For this review, take the finished solid that the model builds, in its own axes (mm). A direction names the side the tool comes from. Coordinates: 2 decimals unless noted, no trailing zeros. Loops run counter-clockwise (first coordinate to the right, second up) from the corner with the lowest first, then second, coordinate; pieces in that order, holes last. Notation, with made-up numbers: (67, 39) -> (73, 39) arc R12 cw to (73, 61) -> close; hole circle Ø4 at (45.25, 34). An arc over 180 degrees is marked (long way). Answer in a Markdown table with one row per item.
from build123d import *

# Parameters (mm, degrees)
BOSS_EXTRUDE1_DEPTH = 5.08
SKETCH2_R           = 2.54
CUT_EXTRUDE1_DEPTH  = 341.814621752
SKETCH3_R           = 2.54
CUT_EXTRUDE2_DEPTH  = 341.814621752
SKETCH4_W           = 3.81
SKETCH4_H           = 37.084
BOSS_EXTRUDE2_DEPTH = 11.43
SKETCH5_W           = 12.7
SKETCH5_H           = 2.54
BOSS_EXTRUDE3_DEPTH = 2.54
BOSS_EXTRUDE4_START = 2.54
SKETCH6_R           = 5.08
SKETCH6_R_2         = 2.54
BOSS_EXTRUDE4_DEPTH = 2.54
SKETCH7_W           = 5.08
SKETCH7_H           = 101.6
BOSS_EXTRUDE5_DEPTH = 57.15
CUT_EXTRUDE3_REACH  = 257.636
SKETCH8_R           = 1.905
SKETCH8_R_2         = 2.54
CUT_EXTRUDE5_REACH  = 257.636
SKETCH10_R          = 2.54
CUT_EXTRUDE7_DEPTH  = 25.4
CUT_EXTRUDE8_DEPTH  = 25.4
CUT_EXTRUDE9_DEPTH  = 346.535703654
SKETCH15_R          = 2.413
SKETCH15_R_2        = 2.54
CUT_EXTRUDE10_DEPTH = 256.636204987


with BuildPart() as part:
    # Sketch1 → Boss-Extrude1 (new body)
    with BuildSketch(Plane(origin=(0, 0, 0), x_dir=(1, 0, 0), z_dir=(0, 1, 0))):
        Polygon((0, 0), (254, 0), (304.8, 76.2), (254, 152.4), (0, 152.4), align=None)
    extrude(amount=BOSS_EXTRUDE1_DEPTH)

    # Sketch2 → Cut-Extrude1 (cut, through all)
    with BuildSketch(Plane(origin=(0, 5.08, 0), x_dir=(1, 0, 0), z_dir=(0, 1, 0))):
        with Locations(Location((76.2, 38.7985, 0), (0, 0, 270))):
            Circle(SKETCH2_R)
        with Locations(Location((167.64, 38.7985, 0), (0, 0, 270))):
            Circle(SKETCH2_R)
        with Locations(Location((167.64, 113.6015, 0), (0, 0, 90))):
            Circle(SKETCH2_R)
        with Locations(Location((76.2, 113.6015, 0), (0, 0, 90))):
            Circle(SKETCH2_R)
    extrude(amount=-CUT_EXTRUDE1_DEPTH, mode=Mode.SUBTRACT)

    # Sketch3 → Cut-Extrude2 (cut, through all)
    with BuildSketch(Plane(origin=(0, 5.08, 0), x_dir=(1, 0, 0), z_dir=(0, 1, 0))):
        with Locations(Location((279.4, 68.58, 0), (0, 0, 270))):
            Circle(SKETCH3_R)
        with Locations(Location((279.4, 83.82, 0), (0, 0, 90))):
            Circle(SKETCH3_R)
    extrude(amount=-CUT_EXTRUDE2_DEPTH, mode=Mode.SUBTRACT)

    # Sketch4 → Boss-Extrude2 (add)
    with BuildSketch(Plane(origin=(0, 5.08, 0), x_dir=(1, 0, 0), z_dir=(0, 1, 0))):
        with Locations((42.545, 18.542)):
            Rectangle(SKETCH4_W, SKETCH4_H)
        with Locations((59.055, 18.542)):
            Rectangle(SKETCH4_W, SKETCH4_H)
        with Locations((59.055, 133.858)):
            Rectangle(SKETCH4_W, SKETCH4_H)
        with Locations((42.545, 133.858)):
            Rectangle(SKETCH4_W, SKETCH4_H)
    extrude(amount=BOSS_EXTRUDE2_DEPTH)

    # Sketch5 → Boss-Extrude3 (add)
    with BuildSketch(Plane(origin=(0, 5.08, 0), x_dir=(1, 0, 0), z_dir=(0, 1, 0))):
        with Locations((50.8, 1.27)):
            Rectangle(SKETCH5_W, SKETCH5_H)
        with Locations((50.8, 151.13)):
            Rectangle(SKETCH5_W, SKETCH5_H)
        with Locations((50.8, 116.586)):
            Rectangle(SKETCH5_W, SKETCH5_H)
        with Locations((50.8, 35.814)):
            Rectangle(SKETCH5_W, SKETCH5_H)
    extrude(amount=BOSS_EXTRUDE3_DEPTH)

    # Sketch6 → Boss-Extrude4 (add)
    # profile 1 of 4: a face of its own
    with BuildSketch(Plane(origin=(0, 5.08, 0), x_dir=(1, 0, 0), z_dir=(0, 1, 0)).offset(BOSS_EXTRUDE4_START)):
        with Locations(Location((76.2, 38.7985, 0), (0, 0, 90))):
            Circle(SKETCH6_R)
        with Locations(Location((76.2, 38.7985, 0), (0, 0, 270))):
            Circle(SKETCH6_R_2, mode=Mode.SUBTRACT)
    # profile 2 of 4: a face of its own
    with BuildSketch(Plane(origin=(0, 5.08, 0), x_dir=(1, 0, 0), z_dir=(0, 1, 0)).offset(BOSS_EXTRUDE4_START)):
        with Locations(Location((167.64, 38.7985, 0), (0, 0, 90))):
            Circle(SKETCH6_R)
        with Locations(Location((167.64, 38.7985, 0), (0, 0, 270))):
            Circle(SKETCH6_R_2, mode=Mode.SUBTRACT)
    # profile 3 of 4: a face of its own
    with BuildSketch(Plane(origin=(0, 5.08, 0), x_dir=(1, 0, 0), z_dir=(0, 1, 0)).offset(BOSS_EXTRUDE4_START)):
        with Locations(Location((167.64, 113.6015, 0), (0, 0, 90))):
            Circle(SKETCH6_R)
        with Locations(Location((167.64, 113.6015, 0), (0, 0, 270))):
            Circle(SKETCH6_R_2, mode=Mode.SUBTRACT)
    # profile 4 of 4: a face of its own
    with BuildSketch(Plane(origin=(0, 5.08, 0), x_dir=(1, 0, 0), z_dir=(0, 1, 0)).offset(BOSS_EXTRUDE4_START)):
        with Locations(Location((76.2, 113.6015, 0), (0, 0, 90))):
            Circle(SKETCH6_R)
        with Locations(Location((76.2, 113.6015, 0), (0, 0, 90))):
            Circle(SKETCH6_R_2, mode=Mode.SUBTRACT)
    extrude(amount=-BOSS_EXTRUDE4_DEPTH)

    # Sketch7 → Boss-Extrude5 (add)
    with BuildSketch(Plane(origin=(0, 5.08, 0), x_dir=(1, 0, 0), z_dir=(0, 1, 0))):
        with Locations((193.04, 76.2)):
            Rectangle(SKETCH7_W, SKETCH7_H)
    extrude(amount=BOSS_EXTRUDE5_DEPTH)

    # Sketch8 → Cut-Extrude3 (cut, up to next)
    with BuildSketch(Plane(origin=(195.58, 0, 0), x_dir=(0, 0, -1), z_dir=(1, 0, 0)), mode=Mode.PRIVATE) as cut_extrude3_sk1:
        with Locations((31.75, 55.88)):
            Circle(SKETCH8_R)
    cut_extrude3_tool1 = extrude(cut_extrude3_sk1.sketch, amount=-CUT_EXTRUDE3_REACH, mode=Mode.PRIVATE) & part.part
    # Sketch8 → Cut-Extrude3 (cut, up to next)
    with BuildSketch(Plane(origin=(195.58, 0, 0), x_dir=(0, 0, -1), z_dir=(1, 0, 0)), mode=Mode.PRIVATE) as cut_extrude3_sk2:
        with Locations((68.834, 55.88)):
            Circle(SKETCH8_R)
    cut_extrude3_tool2 = extrude(cut_extrude3_sk2.sketch, amount=-CUT_EXTRUDE3_REACH, mode=Mode.PRIVATE) & part.part
    # Sketch8 → Cut-Extrude3 (cut, up to next)
    with BuildSketch(Plane(origin=(195.58, 0, 0), x_dir=(0, 0, -1), z_dir=(1, 0, 0)), mode=Mode.PRIVATE) as cut_extrude3_sk3:
        with Locations((50.292, 40.64)):
            Circle(SKETCH8_R_2)
    cut_extrude3_tool3 = extrude(cut_extrude3_sk3.sketch, amount=-CUT_EXTRUDE3_REACH, mode=Mode.PRIVATE) & part.part
    add(cut_extrude3_tool1.solids().sort_by_distance((195.58, 55.88, -31.75))[0], mode=Mode.SUBTRACT)
    add(cut_extrude3_tool2.solids().sort_by_distance((195.58, 55.88, -68.834))[0], mode=Mode.SUBTRACT)
    add(cut_extrude3_tool3.solids().sort_by_distance((195.58, 40.64, -50.292))[0], mode=Mode.SUBTRACT)

    # Sketch10 → Cut-Extrude5 (cut, up to next)
    with BuildSketch(Plane(origin=(195.58, 0, 0), x_dir=(0, 0, -1), z_dir=(1, 0, 0)), mode=Mode.PRIVATE) as cut_extrude5_sk1:
        with Locations((76.2, 16.51)):
            Circle(SKETCH10_R)
    cut_extrude5_tool1 = extrude(cut_extrude5_sk1.sketch, amount=-CUT_EXTRUDE5_REACH, mode=Mode.PRIVATE) & part.part
    add(cut_extrude5_tool1.solids().sort_by_distance((195.58, 16.51, -76.2))[0], mode=Mode.SUBTRACT)

    # Sketch12 → Cut-Extrude7 (cut)
    with BuildSketch(Plane.ZY.offset(-40.64)):
        with BuildLine():
            Line((-20.447, 14.732), (-16.637, 14.732))
            ThreePointArc((-16.637, 14.732), (-15.875, 13.97), (-16.637, 13.208))
            Line((-16.637, 13.208), (-20.447, 13.208))
            ThreePointArc((-20.447, 13.208), (-21.209, 13.97), (-20.447, 14.732))
        make_face()
    extrude(amount=-CUT_EXTRUDE7_DEPTH, mode=Mode.SUBTRACT)

    # Sketch13 → Cut-Extrude8 (cut)
    with BuildSketch(Plane.ZY.offset(-40.64)):
        with BuildLine():
            Line((-135.763, 14.732), (-131.953, 14.732))
            ThreePointArc((-131.953, 14.732), (-131.191, 13.97), (-131.953, 13.208))
            Line((-131.953, 13.208), (-135.763, 13.208))
            ThreePointArc((-135.763, 13.208), (-136.525, 13.97), (-135.763, 14.732))
        make_face()
    extrude(amount=-CUT_EXTRUDE8_DEPTH, mode=Mode.SUBTRACT)

    # Sketch14 → Cut-Extrude9 (cut, through all)
    with BuildSketch(Plane(origin=(0, 5.08, 0), x_dir=(1, 0, 0), z_dir=(0, 1, 0))):
        with BuildLine():
            Line((37.338, 16.637), (37.338, 20.447))
            ThreePointArc((37.338, 20.447), (38.1, 21.209), (38.862, 20.447))
            Line((38.862, 20.447), (38.862, 16.637))
            ThreePointArc((38.862, 16.637), (38.1, 15.875), (37.338, 16.637))
        make_face()
        with BuildLine():
            Line((64.262, 16.637), (64.262, 20.447))
            ThreePointArc((64.262, 20.447), (63.5, 21.209), (62.738, 20.447))
            Line((62.738, 20.447), (62.738, 16.637))
            ThreePointArc((62.738, 16.637), (63.5, 15.875), (64.262, 16.637))
        make_face()
        with BuildLine():
            Line((37.338, 135.763), (37.338, 131.953))
            ThreePointArc((37.338, 131.953), (38.1, 131.191), (38.862, 131.953))
            Line((38.862, 131.953), (38.862, 135.763))
            ThreePointArc((38.862, 135.763), (38.1, 136.525), (37.338, 135.763))
        make_face()
        with BuildLine():
            Line((64.262, 135.763), (64.262, 131.953))
            ThreePointArc((64.262, 131.953), (63.5, 131.191), (62.738, 131.953))
            Line((62.738, 131.953), (62.738, 135.763))
            ThreePointArc((62.738, 135.763), (63.5, 136.525), (64.262, 135.763))
        make_face()
    extrude(amount=-CUT_EXTRUDE9_DEPTH, mode=Mode.SUBTRACT)

    # Sketch15 → Cut-Extrude10 (cut, through all)
    with BuildSketch(Plane(origin=(195.58, 0, 0), x_dir=(0, 0, -1), z_dir=(1, 0, 0))):
        with Locations((83.4136, 55.88)):
            Circle(SKETCH15_R)
        with Locations((119.7864, 55.88)):
            Circle(SKETCH15_R)
        with Locations((101.6, 40.64)):
            Circle(SKETCH15_R_2)
    extrude(amount=-CUT_EXTRUDE10_DEPTH, mode=Mode.SUBTRACT)


solid = part.part
Item 1: The part is to be moulded in two halves that separate along X. For faces 5 (the flat face through (279.756, 2.504, -113.767)), 6 (the flat face through (51, 7, -115.316)), 7 (the flat face through (77, 7.62, -111)), say which applies: +X half, -X half, draft (parallel to the pull), parting line (faces both ways), or undercut.
Worked answers:
| item | result |
|---|---|
| face 5 | +X half |
| face 6 | draft |
| face 7 | undercut |
Item 2: Take a section at A-A, the plane y = 28.5. State the section outline as (x, z) points, and give its area (3 significant figures).
Worked answers:
| item | result |
|---|---|
| outline | (190.5, -127) -> (195.58, -127) -> (195.58, -25.4) -> (190.5, -25.4) -> close |
| area | 516 mm² |
Item 3: For L1, parallel to Z at x = 167.64, y = 6.75; L2, parallel to Y at x = 192.35, z = -31.75 (3 decimals); L3, parallel to X at y = 12, z = -24, list the stretches that pass through material, from the lowest coordinate up.
Worked answers:
| item | result |
|---|---|
| L1 | -118.68 to -116.14, -111.06 to -108.52, -43.88 to -41.34, -36.26 to -33.72 |
| L2 | 0 to 53.975, 57.785 to 62.23 |
| L3 | 40.64 to 44.45, 57.15 to 60.96 |
Item 4: Insertion check: pin 1 (8 mm diameter, centred on x = 229, z = -77.5, fed in from +Y); pin 2 (5 mm diameter, centred on y = 48.5, z = -124, fed in from -X); pin 3 (12.5 mm diameter, centred on y = 13.5, z = -13.5, fed in from -X). Each pin has a flat end and moves straight along its axis. Give the tip position at first contact, or say it passes through.
Worked answers:
| item | result |
|---|---|
| pin 1 | y = 5.08 |
| pin 2 | x = 190.5 |
| pin 3 | x = 40.64 |
Item 5: Take a section at B-B, the plane x = 183.5. State the section outline as (y, z) points.
Worked answers:
| item | result |
|---|---|
| outline | (0, -152.4) -> (5.08, -152.4) -> (5.08, 0) -> (0, 0) -> close |
Item 6: For faces 1 (the flat face through (195.58, 33, -75)), 2 (the flat face through (60.96, 11, -134)), 3 (the cylindrical face through (172.6, 6.4, -37.7)), 4 (the flat face through (101, 4, -152.4)), list the 3-axis set-ups (+Z, -Z, +X, -X, +Y, -Y) from which the entire face can be reached by the end or side of a thin tool; tool diameter is ignored.
Worked answers:
| item | result |
|---|---|
| face 1 | +Z, -Z, +X, +Y |
| face 2 | +Z, -Z, +Y |
| face 3 | +Y |
| face 4 | -Z, +X, -X, +Y, -Y |
Item 7: Take a section at C-C, the plane z = -140. State the section outline as (x, y) points, and give its area (3 significant figures).
Worked answers:
| item | result |
|---|---|
| outline | (0, 0) -> (262.27, 0) -> (262.27, 5.08) -> (60.96, 5.08) -> (60.96, 16.51) -> (57.15, 16.51) -> (57.15, 5.08) -> (44.45, 5.08) -> (44.45, 16.51) -> (40.64, 16.51) -> (40.64, 5.08) -> (0, 5.08) -> close |
| area | 1,420 mm² |
